Autodesk Inventor part; units mm, degrees
ref_plane "Work Plane1" through (-1275, 0, -1250) normal (-1, 0, 0) x (0, 0, 1)
ref_plane "Work Plane2" through (0, 0, -625) normal (0, 0, -1) x (-1, 0, 0)
ref_plane "YZ Plane" through (0, 0, 0) normal (1, 0, 0) x (0, 1, 0)
sketch "Sketch1" plane through (0, 0, 0) normal (0, 1, 0) x (-1, 0, 0)
  line L0 (0, 0) -> (2550, 0)
  line L1 (2550, 0) -> (2550, -1250)
  line L2 (2550, -1250) -> (0, -1250)
  line L3 (0, -1250) -> (0, 0)
  dimension "d0" = 1250
  dimension "d1" = 2550
extrude "Extrusion1" add sketch "Sketch1" along normal blind 20
sketch "Sketch2" plane through (0, 20, 0) normal (0, 1, 0) x (1, 0, 0)
  line L0 (-2550, 0) -> (0, 0)
  line L1 (0, 0) -> (0, 1250)
  line L2 (0, 1250) -> (-2550, 1250)
  line L3 (-2550, 1250) -> (-2550, 0)
  circle A0 centre (-2500, 1100) radius 25
  dimension "d4" = 50
  dimension "d5" = 1250
  dimension "d6" = 150
  dimension "d7" = 50
ref_plane "Work Plane1" through (-1275, 0, -1250) normal (-1, 0, 0) x (0, 0, 1)
ref_plane "Work Plane2" through (0, 0, -625) normal (0, 0, -1) x (-1, 0, 0)
extrude "Extrusion2" cut sketch "Sketch2" against normal blind 10 contours A0
mirror "Mirror1" about plane through (0, 0, -625) normal (0, 0, -1) of "Extrusion2"
mirror "Mirror2" about plane through (-1275, 0, -1250) normal (-1, 0, 0) of "Extrusion2", "Mirror1"
properties part number "Led Plater" material "Aluminum 6061"
Check sheet for the modelled part. Datum: model origin and axes. Units: mm. A direction names the side the tool comes from. Give positions to 0.01 mm unless a question says otherwise; leave off trailing zeros. Write each loop counter-clockwise with the first axis right and the second up, starting at its lowest first coordinate (ties: lowest second). Pieces come first, ordered by that corner, then holes. Notation, with made-up numbers: M 9.25,57.5 L 40.25,57.5 A18 cw 40.25,83.5 Z; hole C 15,73 d7. An arc over 180 degrees is marked long. Use one line per item in the form item = value.
(1) Section check B-B on z = -1100. Record the boundary of the cut face in (x, y).
Answer block:
outline = M -2550,0 L 0,0 L 0,20 L -25,20 L -25,10 L -75,10 L -75,20 L -2475,20 L -2475,10 L -2525,10 L -2525,20 L -2550,20 Z
(2) Section check A-A on x = -50. Record the boundary of the cut face in (y, z).
Answer block:
outline = M 0,-1250 L 20,-1250 L 20,-1125 L 10,-1125 L 10,-1075 L 20,-1075 L 20,-175 L 10,-175 L 10,-125 L 20,-125 L 20,0 L 0,0 Z
(3) Tool access check on faces 1 (the flat face through (-2500, 10, -1100)), 2 (the flat face through (-1257, 0, -616)). Record the directions out of +Z, -Z, +X, -X, +Y, -Y that give a thin tool (end or side, any length) a straight path to the whole face; none if there is none.
Answer block:
face_1 = +Y
face_2 = +Z, -Z, +X, -X, -Y
(4) Draft check along Z on faces 3 (the cylindrical face through (-46.745, 15.07, -125.213)), 4 (the flat face through (-1257, 20, -616)). Enter one of: pulls with the +Z half, pulls with the -Z half, needs draft (parallel to the pull), parting line crosses it, or undercut.
Answer block:
face_3 = undercut
face_4 = needs draft
(5) Material ranges on line 1 along Z through (x, y) = (-50, 14.5); line 2 along X through (y, z) = (17.75, -1100), recorded low to high.
Answer block:
line_1 = -1250 to -1125, -1075 to -175, -125 to 0
line_2 = -2550 to -2525, -2475 to -75, -25 to 0
(6) Depth check by flat-ended pin: P1, Ø15, axis at x = -2505.5, z = -150.5, coming from the +Y side. Enter the tip coordinate at first touch or a pass-through.
Answer block:
P1 = 10
